For this review, take the finished solid that the model builds, in its own axes (mm). Face numbers are marked on the shaded views. A direction names the side the tool comes from. Round coordinates to 2 decimals unless told otherwise and drop trailing zeros. Order: outer loops, then holes, each group sorted by start corner. A loop starts at its lowest first (then second) coordinate and runs counter-clockwise, first axis right, second up. Notation, with made-up numbers: M -1,-17 L 18,-17 A21 ccw 18,3 Z; hole C 37.25,57.5 d8. An arc over 180 degrees is marked long. Write item = value, one per line. Start each with the question number.
from build123d import *

# Parameters (mm, degrees)
SKETCH_1_R      = 1.5
EXTRUDE_1_DEPTH = 48
EXTRUDE_START   = -12
SKETCH_2_R      = 2.5
SKETCH_2_R_2    = 1.5
EXTRUDE_2_DEPTH = 12
EXTRUDE_START_2 = 24
SKETCH_3_R      = 2
SKETCH_3_R_2    = 1.5
EXTRUDE_3_DEPTH = 5.5


with BuildPart() as part:
    # 草图1 → 凸台-拉伸1 (new body)
    with BuildSketch(Plane(origin=(0, 0, 0), x_dir=(0, 0, -1), z_dir=(1, 0, 0))):
        Circle(SKETCH_1_R)
    extrude(amount=EXTRUDE_1_DEPTH)

    # 草图2 → 凸台-拉伸2 (add)
    with BuildSketch(Plane.ZY.offset(EXTRUDE_START)):
        Circle(SKETCH_2_R)
        Circle(SKETCH_2_R_2, mode=Mode.SUBTRACT)
    extrude(amount=-EXTRUDE_2_DEPTH)

    # 草图3 → 凸台-拉伸3 (add)
    with BuildSketch(Plane(origin=(0, 0, 0), x_dir=(0, 0, -1), z_dir=(1, 0, 0)).offset(EXTRUDE_START_2)):
        with Locations(Location((0, 0, 0), (0, 0, 180))):
            Circle(SKETCH_3_R)
        with Locations(Location((0, 0, 0), (0, 0, 180))):
            Circle(SKETCH_3_R_2, mode=Mode.SUBTRACT)
    extrude(amount=EXTRUDE_3_DEPTH)


solid = part.part
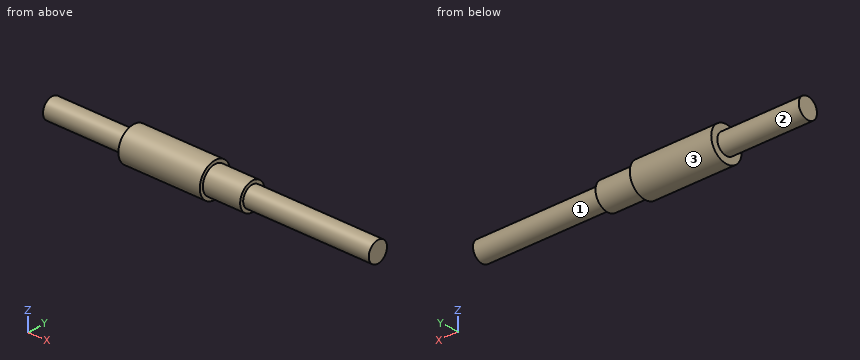
(1) For line 1 along X through (y, z) = (1.55, -0.95); line 2 along X through (y, z) = (-1.95, -1.05); line 3 along Z through (x, y) = (40.5, 0), list the stretches that pass through material, from the lowest coordinate up.
(2) We need section A-A, the plane y = 0. Write out the cut boundary in (x, z), then the cut area to 4 significant figures.
(3) Insertion check: pin 1 (1 mm diameter, centred on y = 0, z = 1.5, fed in from -X). The pin has a flat end and moves straight along its axis. Give the tip position at first contact, or say it passes through.
(4) For the marked faces 1, 2 and 3, list the 3-axis set-ups (+Z, -Z, +X, -X, +Y, -Y) from which the entire face can be reached by the end or side of a thin tool; tool diameter is ignored.
(5) We need section D-D, the plane x = 11. Write out the cut boundary in (y, z), then the cut area to 3 significant figures.
(6) We need section C-C, the plane x = 28. Write out the cut boundary in (y, z).
Values:
q1.line_1 = 12 to 29.5
q1.line_2 = 12 to 24
q1.line_3 = -1.5 to 1.5
q2.outline = M 0,-1.5 L 12,-1.5 L 12,-2.5 L 24,-2.5 L 24,-2 L 29.5,-2 L 29.5,-1.5 L 48,-1.5 L 48,1.5 L 29.5,1.5 L 29.5,2 L 24,2 L 24,2.5 L 12,2.5 L 12,1.5 L 0,1.5 Z
q2.area = 173.5 mm²
q3.pin_1 = 0
q4.face_1 = +X
q4.face_2 = -X
q4.face_3 = +X, -X
q5.outline = C 0,0 d3
q5.area = 7.07 mm²
q6.outline = C 0,0 d4
